from build123d import *

# Parameters (mm, degrees)
SKETCH_1_R      = 10
SKETCH_1_R_2    = 8.1
EXTRUDE_1_DEPTH = 10
SKETCH_2_R      = 8.1
SKETCH_2_R_2    = 6.6
EXTRUDE_2_DEPTH = 10
SKETCH_3_W      = 20
SKETCH_3_H      = 20
EXTRUDE_3_DEPTH = 20
SKETCH1_W       = 32.202662478
SKETCH1_H       = 25
EXTRUDE1_DEPTH  = 10
CHAMFER1_SIZE   = 1


with BuildPart() as part:
    # 스케치1 → 보스-돌출1 (new, symmetric)
    # profile 1 of 2: a face of its own
    with BuildSketch(Plane.XY):
        Circle(SKETCH_1_R)
        Circle(SKETCH_1_R_2, mode=Mode.SUBTRACT)
    # profile 2 of 2: a face of its own
    with BuildSketch(Plane.XY):
        with BuildLine():
            Line((-9.396926208, 3.420201433), (-16.101331239, -15))
            Line((-16.101331239, -15), (16.101331239, -15))
            Line((16.101331239, -15), (9.396926208, 3.420201433))
            ThreePointArc((9.396926208, 3.420201433), (9.84807753, 1.736481777), (10, 0))
            ThreePointArc((10, 0), (-1.736481777, -9.84807753), (-9.396926208, 3.420201433))
        make_face()
    extrude(amount=EXTRUDE_1_DEPTH, both=True)

    # 스케치2 → 보스-돌출2 (add)
    with BuildSketch(Plane.XY):
        Circle(SKETCH_2_R)
        Circle(SKETCH_2_R_2, mode=Mode.SUBTRACT)
    extrude(amount=EXTRUDE_2_DEPTH)

    # 스케치3 → 보스-돌출3 (add)
    with BuildSketch(Plane.XZ.offset(15)):
        Rectangle(SKETCH_3_W, SKETCH_3_H)
    extrude(amount=EXTRUDE_3_DEPTH)

    # Sketch1 → Extrude1 (cut)
    with BuildSketch(Plane.XY.offset(10)):
        with Locations((0, -2.5)):
            Rectangle(SKETCH1_W, SKETCH1_H)
    extrude(amount=-EXTRUDE1_DEPTH, mode=Mode.SUBTRACT)

    # Chamfer1
    chamfer1_edges = [part.edges().sort_by_distance(p)[0] for p in [
        (0, -15, 0),
    ]]
    chamfer(chamfer1_edges, length=CHAMFER1_SIZE)


solid = part.part
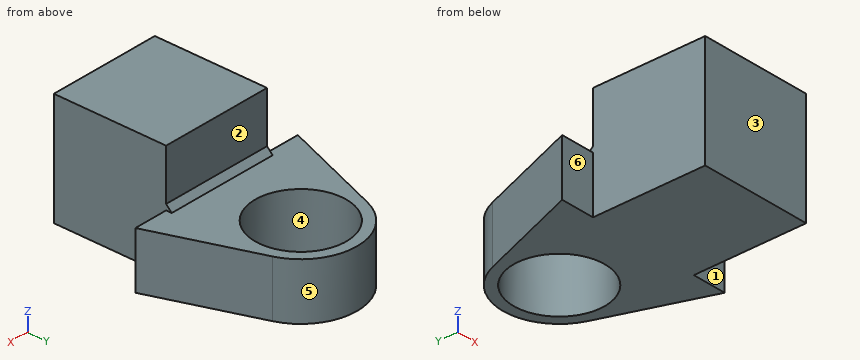
Can you work these out from the model? Positions are in its coordinate system, mm. Face numbers are marked on the shaded views. A direction names the side the tool comes from. Give positions to 0.01 mm unless a question says otherwise; leave off trailing zeros. Loops run counter-clockwise (first coordinate to the right, second up) from the corner with the lowest first, then second, coordinate; pieces in that order, holes last. Notation, with made-up numbers: M 58,39.25 L 63,39.25 A20 cw 63,64.25 Z; hole C 15.25,47.5 d3. An arc over 180 degrees is marked long. One line per item, written item: value.
1) Imagine slicing it at B-B on y = 0. Write out the boundary of the cut face in (x, z), and give its area (3 significant figures).
Geometry check:
outline: M -10.64,-10 L -8.1,-10 L -8.1,0 L -10.64,0 Z; M 8.1,-10 L 10.64,-10 L 10.64,0 L 8.1,0 Z
area: 50.8 mm²
2) Imagine slicing it at D-D on y = -21. Write out the boundary of the cut face in (x, z).
Geometry check:
outline: M -10,-10 L 10,-10 L 10,10 L -10,10 Z
3) Imagine slicing it at C-C on z = -5.25. Write out the boundary of the cut face in (x, y), and give its area (3 significant figures).
Geometry check:
outline: M -16.1,-15 L -10,-15 L -10,-35 L 10,-35 L 10,-15 L 16.1,-15 L 9.4,3.42 A10 ccw -9.4,3.42 Z; hole C 0,0 d16.2
area: 754 mm²
4) I'm going to push flat-ended pins straight in: pin 1 (12 mm diameter, centred on y = -15.5, z = 6.5, fed in from -X); pin 2 (12.5 mm diameter, centred on x = 2, y = -0.5, fed in from +Z); pin 3 (1.8 mm diameter, centred on x = -14, z = -3, fed in from -Y); pin 4 (1 mm diameter, centred on x = -11, z = 5, fed in from +Y). Where does each tip first touch, or does it pass through?
Geometry check:
pin 1: stops at x = -10
pin 2: stops at z = 0
pin 3: stops at y = -15
pin 4: passes through
5) Please list where these lines run through material, in increasing order: line 1 (Y direction, x = 0, z = -3.5); line 2 (Z direction, x = 5.5, y = -10); line 3 (X direction, y = -1.5, z = -8.5).
Geometry check:
line 1: y = -35 to -8.1, 8.1 to 10
line 2: z = -10 to 0
line 3: x = -11.19 to -7.96, 7.96 to 11.19
6) On a 3-axis mill with a long thin cutter (end or side, diameter ignored), from which of +Z, -Z, +X, -X, +Y, -Y can I reach the whole of each face in a straight line? I mean the marked faces 1, 2 and 3. Say none if no direction works.
Geometry check:
face 1: +Z, -Z, +X, -Y
face 2: +Z, +X, -X, +Y
face 3: +Z, -Z, +X, -X, -Y
7) Thinking about a two-plate mould opening in X: for the marked faces 4, 5 and 6, which applies, +X half, -X half, draft (parallel to the pull), parting line (faces both ways), or undercut?
Geometry check:
face 4: undercut
face 5: parting line
face 6: draft
8) Imagine slicing it at A-A on x = 0. Write out the boundary of the cut face in (y, z), and give its area (4 significant figures).
Geometry check:
outline: M -35,-10 L -8.1,-10 L -8.1,0 L -14,0 L -15,1 L -15,10 L -35,10 Z; M 8.1,-10 L 10,-10 L 10,0 L 8.1,0 Z
area: 488.5 mm²
